Autodesk Inventor part; units mm, degrees
ref_plane "YZ Plane" through (0, 0, 0) normal (1, 0, 0) x (0, 1, 0)
ref_plane "XZ Plane" through (0, 0, 0) normal (0, 1, 0) x (-1, 0, 0)
ref_plane "XY Plane" through (0, 0, 0) normal (0, 0, 1) x (1, 0, 0)
sketch "Sketch1" plane through (0, 0, 0) normal (0, 1, 0) x (-1, 0, 0)
  line L0 (-30, -40) -> (-30, 40)
  line L1 (-30, 40) -> (30, 40)
  line L2 (30, 40) -> (30, -40)
  line L3 (30, -40) -> (-30, -40)
  line L4 (-30, -40) -> (30, 40) construction
  line L5 (-30, 40) -> (30, -40) construction
  point P0 (0, 0)
  dimension "d0" = 80
  dimension "d1" = 60
extrude "Extrusion1" add sketch "Sketch1" along normal blind 5
sketch "Sketch2" plane through (0, 5, 0) normal (0, 1, 0) x (1, 0, 0)
  circle A0 centre (-5.5, -37.5) radius 1
  circle A1 centre (5.5, -37.5) radius 1
  line L0 (-30, -40) -> (30, -40)
  line L1 (30, -40) -> (30, 40)
  point P0 (0, 0)
  dimension "d4" = 2
  dimension "d5" = 2
  dimension "d6" = 11
  dimension "d7" = 2.5
  dimension "d8" = 2.5
  dimension "d9" = 24.5
extrude "Extrusion2" cut sketch "Sketch2" against normal blind 4
sketch "Sketch3" plane through (0, 5, 0) normal (0, 1, 0) x (1, 0, 0)
  line L0 (30, -40) -> (30, 40)
  line L1 (30, -40) -> (0, -40)
  line L2 (-30, -40) -> (30, -40)
  line L3 (0, -40) -> (0, 2.107)
  line L4 (0, 2.107) -> (-6, 2.107)
  line L5 (-6, 2.107) -> (-6, 8.207)
  line L6 (-6, 8.207) -> (16.75, 8.207)
  line L7 (16.75, 8.207) -> (16.75, -3.993)
  line L8 (16.75, -3.993) -> (-6, -3.993)
  line L9 (-6, -3.993) -> (-6, 8.207)
  point P0 (0, 0)
  dimension "d12" = 42.107
  dimension "d13" = 6
  dimension "d14" = 6.1
  dimension "d15" = 22.75
  dimension "d16" = 12.2
extrude "Extrusion3" cut sketch "Sketch3" against normal blind 3.915
sketch "Sketch4" plane through (30, 0, 40) normal (1, 0, 0) x (0, 0, -1)
  line L0 (0, 0) -> (80, 0)
  line L1 (0, 5) -> (80, 5)
  line L2 (80, 5) -> (80, 0)
  line L3 (80, 0) -> (0, 0)
  line L4 (0, 0) -> (0, 5)
  point P0 (40, 0)
extrude "Extrusion4" add sketch "Sketch4" along normal blind 20
sketch "Sketch5" plane through (-30, 0, -40) normal (0, 0, -1) x (-1, 0, 0)
  line L0 (0, 5) -> (-80, 5)
  line L1 (0, 0) -> (0, 5)
  line L2 (-80, 5) -> (0, 5)
  line L3 (0, 5) -> (0, 0)
  line L4 (0, 0) -> (-80, 0)
  line L5 (-80, 0) -> (-80, 5)
  point P0 (-30, 0)
extrude "Extrusion5" add sketch "Sketch5" along normal blind 10
sketch "Sketch6" plane through (0, 5, 0) normal (0, 1, 0) x (1, 0, 0)
  line L0 (-30, -40) -> (-30, 50)
  line L1 (-30, -40) -> (0, -40)
  line L2 (-30, -40) -> (50, -40)
  line L3 (0, -40) -> (0, 32.107)
  line L4 (0, 32.107) -> (22.5, 32.107)
  line L5 (22.5, 32.107) -> (16.5, 32.107)
  line L6 (16.5, 32.107) -> (16.5, 38.207)
  line L7 (16.5, 38.207) -> (39.25, 38.207)
  line L8 (39.25, 38.207) -> (39.25, 26.007)
  line L9 (39.25, 26.007) -> (16.5, 26.007)
  line L10 (16.5, 26.007) -> (16.5, 38.207)
  point P0 (0, 0)
  dimension "d23" = 30
  dimension "d24" = 72.107
  dimension "d25" = 22.5
  dimension "d26" = 6
  dimension "d27" = 6.1
  dimension "d28" = 22.75
  dimension "d29" = 12.2
extrude "Extrusion6" add sketch "Sketch6" along normal blind 18.52
sketch "Sketch7" plane through (0, 5, 0) normal (0, 1, 0) x (1, 0, 0)
  line L0 (16.75, 8.207) -> (16.75, -3.993)
  line L1 (16.75, -3.993) -> (21.625, -3.993)
  line L2 (21.625, -3.993) -> (21.625, 8.207)
  line L3 (21.625, 8.207) -> (16.75, 8.207)
  line L4 (16.75, 8.207) -> (16.75, -3.993)
  line L5 (-6, -3.993) -> (-6, 8.207)
  line L6 (-6, -3.993) -> (-10.875, -3.993)
  line L7 (-10.875, -3.993) -> (-10.875, 8.207)
  line L8 (-10.875, 8.207) -> (-6, 8.207)
  line L9 (-6, 8.207) -> (-6, -3.993)
  point P0 (0, 0)
  dimension "d32" = 4.875
  dimension "d33" = 4.875
  dimension "d34" = 12.2
extrude "Extrusion7" add sketch "Sketch7" along normal blind 14.135
sketch "Sketch8" plane through (-6, 1.085, 3.993) normal (1, 0, 0) x (0, 0, -1)
  line L0 (0, 0) -> (12.2, 0)
  line L1 (6.1, 0) -> (6.1, 3.8)
  line L2 (6.1, 3.8) -> (11.1, 3.8)
  line L3 (11.1, 3.8) -> (1.1, 3.8)
  line L4 (1.1, 3.8) -> (1.1, 6.8)
  line L5 (1.1, 6.8) -> (11.1, 6.8)
  line L6 (11.1, 6.8) -> (11.1, 3.8)
  point P0 (3.993, -1.085)
  dimension "d37" = 3.8
  dimension "d38" = 5
  dimension "d39" = 10
  dimension "d40" = 3
extrude "Extrusion8" cut sketch "Sketch8" against normal blind 12
sketch "Sketch9" plane through (0, 5, 0) normal (0, 1, 0) x (1, 0, 0)
  line L0 (16.5, 26.007) -> (16.5, 38.207)
  line L1 (16.5, 26.007) -> (11.625, 26.007)
  line L2 (11.625, 26.007) -> (11.625, 38.207)
  line L3 (11.625, 38.207) -> (16.5, 38.207)
  line L4 (16.5, 38.207) -> (16.5, 26.007)
  line L5 (39.25, 26.007) -> (16.5, 26.007)
  line L6 (39.25, 26.007) -> (44.125, 26.007)
  line L7 (44.125, 26.007) -> (44.125, 38.207)
  line L8 (44.125, 38.207) -> (39.25, 38.207)
  line L9 (39.25, 38.207) -> (39.25, 26.007)
  point P0 (0, 0)
  dimension "d43" = 4.875
  dimension "d44" = 12.2
  dimension "d45" = 4.875
  dimension "d46" = 12.2
extrude "Extrusion9" add sketch "Sketch9" along normal blind 36.57
sketch "Sketch10" plane through (16.5, 23.52, -38.207) normal (1, 0, 0) x (0, 0, -1)
  line L0 (0, 0) -> (-12.2, 0)
  line L1 (-6.1, 0) -> (-6.1, 3.8)
  line L2 (-6.1, 3.8) -> (-1.1, 3.8)
  line L3 (-1.1, 3.8) -> (-11.1, 3.8)
  line L4 (-11.1, 3.8) -> (-11.1, 6.8)
  line L5 (-11.1, 6.8) -> (-1.1, 6.8)
  line L6 (-1.1, 6.8) -> (-1.1, 3.8)
  point P0 (-38.207, -23.52)
  point P1 (-6.1, 3.8)
  dimension "d49" = 3.8
  dimension "d50" = 5
  dimension "d51" = 10
  dimension "d52" = 3
extrude "Extrusion10" cut sketch "Sketch10" against normal up to surface (4.875 mm away)
fillet "Fillet1" radius 2 8 edges at (21.625, 12.0675, 3.993) (21.625, 12.0675, -8.207) (-10.875, 12.0675, 3.993) (-10.875, 12.0675, -8.207) (11.625, 23.285, -38.207) (11.625, 23.285, -26.007) (44.125, 23.285, -26.007) (44.125, 23.285, -38.207)
properties part number "Base"
Can you work these out from the model? Positions are in its coordinate system, mm. A direction names the side the tool comes from. Give positions to 0.01 mm unless a question says otherwise; leave off trailing zeros. Order: outer loops, then holes, each group sorted by start corner. A loop starts at its lowest first (then second) coordinate and runs counter-clockwise, first axis right, second up. Notation, with made-up numbers: (-7.75, 6.25) - (48.25, 6.25) arc R20 ccw to (48.25, 10.25) - close; hole circle Ø5 at (-2, 41.25). An arc over 180 degrees is marked (long way). Write each question's results on one line, items separated by ' | '.
1) If we mould it in two halves opening along X, with no side actions, what happens to faces 6 (the face through (5, 1.085, -2)), 7 (the face through (18, 12, 3.993)), 8 (the face through (11.625, 16, -32))? For each: pulls with the +X half, pulls with the -X half, needs draft (parallel to the pull), parting line crosses it, or undercut.
Final values:
face 6: undercut | face 7: needs draft | face 8: pulls with the -X half
2) Suppose I cut it at B-B, the plane y = 16.5. Write out the boundary of the cut face in (x, z) (3 decimals).
Final values:
outline: (-10.875, -6.207) arc R2 ccw to (-8.875, -8.207) - (-6, -8.207) - (-6, 3.993) - (-8.875, 3.993) arc R2 ccw to (-10.875, 1.993) - close; (11.625, -36.207) arc R2 ccw to (13.625, -38.207) - (42.125, -38.207) arc R2 ccw to (44.125, -36.207) - (44.125, -28.007) arc R2 ccw to (42.125, -26.007) - (13.625, -26.007) arc R2 ccw to (11.625, -28.007) - close; (16.75, -8.207) - (19.625, -8.207) arc R2 ccw to (21.625, -6.207) - (21.625, 1.993) arc R2 ccw to (19.625, 3.993) - (16.75, 3.993) - close
3) I'm going to push flat-ended pins straight in: pin 1 Ø10 at (x, z) = (26, -5.5) entering from +Y (3 decimals); pin 2 Ø14 at (x, y) = (22, 15.5) entering from +Z; pin 3 Ø2.5 at (x, y) = (14.5, 29) entering from +Z. Where does each tip first touch, or does it pass through?
Final values:
pin 1: stops at y = 19.135 | pin 2: stops at z = 3.99 | pin 3: stops at z = -26.01
4) Suppose I cut it at C-C, the plane z = -31.5. Write out the boundary of the cut face in (x, y) (3 decimals).
Final values:
outline: (-30, 0) - (50, 0) - (50, 5) - (44.125, 5) - (44.125, 41.57) - (39.25, 41.57) - (39.25, 23.52) - (16.5, 23.52) - (16.5, 27.32) - (11.625, 27.32) - (11.625, 5) - (-30, 5) - close; (11.625, 30.32) - (16.5, 30.32) - (16.5, 41.57) - (11.625, 41.57) - close
5) Please list where these lines run through material, in increasing order: line 1 along X through (y, z) = (4.2, 37.5); line 2 along Z through (x, y) = (-5.5, 4.2); line 3 along Y through (x, z) = (-9, 2.5) (3 decimals). Write a range as [from, to].
Final values:
line 1: x = [-30, -6.5], [-4.5, 4.5], [6.5, 50] | line 2: z = [-50, -8.21], [3.99, 36.5], [38.5, 40] | line 3: y = [0, 4.885], [7.885, 19.135]
6) On a 3-axis mill with a long thin cutter (end or side, diameter ignored), from which of +Z, -Z, +X, -X, +Y, -Y can I reach the whole of each face in a straight line? I mean faces 1 (the face through (-7, 12, 3.993)), 2 (the face through (16.5, 32, -32)), 3 (the face through (5.37, 3.03, 36.51)), 4 (the face through (14, 29, -37.107)), 5 (the face through (18, 12, -8.207)). Say none if no direction works.
Final values:
face 1: +Z, +X, -X, +Y | face 2: +Z, -Z, +Y | face 3: +Y | face 4: -X | face 5: +X, -X, +Y
7) Suppose I cut it at A-A, the plane y = 33. Write out the boundary of the cut face in (x, z) (3 decimals), then the cut area to 3 significant figures.
Final values:
outline: (11.625, -36.207) arc R2 ccw to (13.625, -38.207) - (16.5, -38.207) - (16.5, -26.007) - (13.625, -26.007) arc R2 ccw to (11.625, -28.007) - close; (39.25, -38.207) - (42.125, -38.207) arc R2 ccw to (44.125, -36.207) - (44.125, -28.007) arc R2 ccw to (42.125, -26.007) - (39.25, -26.007) - close | area: 116 mm^2
8) Suppose I cut it at D-D, the plane x = 29.5. Write out the boundary of the cut face in (y, z).
Final values:
outline: (0, -50) - (5, -50) - (5, -38.21) - (23.52, -38.21) - (23.52, -26.01) - (5, -26.01) - (5, 40) - (0, 40) - close
